Can you work these out from the model? Positions are in its coordinate system, mm. A direction names the side the tool comes from. Round coordinates to 2 decimals unless told otherwise and drop trailing zeros.
from build123d import *

# Parameters (mm, degrees)
SKETCH1_W           = 38
SKETCH1_H           = 70
BOSS_EXTRUDE1_DEPTH = 5
SKETCH2_R           = 1.65
CUT_EXTRUDE1_DEPTH  = 134.018795664
FILLET1_R           = 3
FILLET2_DEPTH       = 5
SKETCH3_W           = 188
SKETCH3_H           = 3
BOSS_EXTRUDE2_DEPTH = 8
SKETCH4_W           = 5
SKETCH4_H           = 39
BOSS_EXTRUDE3_DEPTH = 8
BOSS_EXTRUDE4_DEPTH = 5
FILLET3_SIZE        = 40
FILLET3_SIZE_2      = 10
FILLET4_SIZE        = 40
FILLET4_SIZE_2      = 10
CUT_EXTRUDE2_DEPTH  = 134.165310942


with BuildPart() as part:
    # Sketch1 → Boss-Extrude1 (new body)
    with BuildSketch(Plane.XY):
        with Locations((19, -35)):
            Rectangle(SKETCH1_W, SKETCH1_H)
        Polygon((-75, 15), (-75, 0), (0, 0), (38, 0), (113, 0), (113, 15), align=None)
    extrude(amount=BOSS_EXTRUDE1_DEPTH)

    # Sketch2 → Cut-Extrude1 (cut, through all)
    with BuildSketch(Plane.XY.offset(5)):
        with Locations((34, -66)):
            Circle(SKETCH2_R)
        with Locations((4, -66)):
            Circle(SKETCH2_R)
        with Locations((4, -40)):
            Circle(SKETCH2_R)
        with Locations((34, -40)):
            Circle(SKETCH2_R)
    extrude(amount=-CUT_EXTRUDE1_DEPTH, mode=Mode.SUBTRACT)

    # Fillet1
    fillet1_edges = [part.edges().sort_by_distance(p)[0] for p in [
        (38, -70, 2.5),
        (0, -70, 2.5),
    ]]
    fillet(fillet1_edges, radius=FILLET1_R)

    # Fillet2: read off the stored shape, not the designer's step
    # Fillet2 outline → Fillet2 (add)
    with BuildSketch(Plane.XY):
        with BuildLine():
            add(Edge.make_bspline(
                [(58, 0), (38, 0), (38, -20)],
                knots=[0, 0, 0, 1, 1, 1], degree=2, weights=[1, 0.052631579, 1]))
            Line((58, 0), (38, 0))
            Line((38, 0), (38, -20))
        make_face()
        with BuildLine():
            Line((0, 0), (-20, 0))
            add(Edge.make_bspline(
                [(-20, 0), (0, 0), (0, -20)],
                knots=[0, 0, 0, 1, 1, 1], degree=2, weights=[1, 0.052631579, 1]))
            Line((0, -20), (0, 0))
        make_face()
    extrude(amount=FILLET2_DEPTH)

    # Sketch3 → Boss-Extrude2 (add)
    with BuildSketch(Plane.XY.offset(5)):
        with Locations((19, 4.5)):
            Rectangle(SKETCH3_W, SKETCH3_H)
    extrude(amount=BOSS_EXTRUDE2_DEPTH)

    # Sketch4 → Boss-Extrude3 (add)
    with BuildSketch(Plane.XY.offset(5)):
        with Locations((19, -16.5)):
            Rectangle(SKETCH4_W, SKETCH4_H)
    extrude(amount=BOSS_EXTRUDE3_DEPTH)

    # Sketch5 → Boss-Extrude4 (add)
    with BuildSketch(Plane.XY.offset(5)):
        Polygon((-52, 0), (-57.902965871, 0), (-60, 0), (0, -30), (0, -25), align=None)
        Polygon((38, -30), (98, 0), (90, 0), (38, -25), align=None)
    extrude(amount=-BOSS_EXTRUDE4_DEPTH)

    # Fillet3
    # a fillet whose section is not a circle: 40, 10 mm, written as the material it takes off along each edge
    with BuildSketch(Plane(origin=(-75, 15, -100), x_dir=(1, 0, 0), z_dir=(0, 0, 1))) as fillet3_piece_1:
        with BuildLine():
            Bezier((FILLET3_SIZE, 0), (0, 0), (0, -FILLET3_SIZE_2), weights=[1, 0.707106781, 1])
            Line((0, -FILLET3_SIZE_2), (0, 0))
            Line((0, 0), (FILLET3_SIZE, 0))
        make_face()
    extrude(amount=205, mode=Mode.SUBTRACT)

    # Fillet4
    # a fillet whose section is not a circle: 40, 10 mm, written as the material it takes off along each edge
    with BuildSketch(Plane(origin=(113, 15, -100), x_dir=(-1, 0, 0), z_dir=(0, 0, 1))) as fillet4_piece_1:
        with BuildLine():
            Bezier((FILLET4_SIZE, 0), (0, 0), (0, FILLET4_SIZE_2), weights=[1, 0.707106781, 1])
            Line((0, FILLET4_SIZE_2), (0, 0))
            Line((0, 0), (FILLET4_SIZE, 0))
        make_face()
    extrude(amount=205, mode=Mode.SUBTRACT)

    # Sketch6 → Cut-Extrude2 (cut, through all)
    with BuildSketch(Plane.XY.offset(5)):
        with BuildLine():
            Line((3.671572875, -13.862410437), (-3.399494937, -6.791342626))
            ThreePointArc((-3.399494937, -6.791342626), (-3.399494937, -1.134488376), (2.257359313, -1.134488376))
            Line((2.257359313, -1.134488376), (9.328427125, -8.205556188))
            ThreePointArc((9.328427125, -8.205556188), (9.328427125, -13.862410437), (3.671572875, -13.862410437))
        make_face()
        with BuildLine():
            Line((28.671572875, -8.445013015), (35.742640687, -1.373945203))
            ThreePointArc((35.742640687, -1.373945203), (41.399494937, -1.373945203), (41.399494937, -7.030799453))
            Line((41.399494937, -7.030799453), (34.328427125, -14.101867265))
            ThreePointArc((34.328427125, -14.101867265), (28.671572875, -14.101867265), (28.671572875, -8.445013015))
        make_face()
    extrude(amount=-CUT_EXTRUDE2_DEPTH, mode=Mode.SUBTRACT)


solid = part.part
(1) If I drill on line 1 (X direction, y = -66, z = 3.7); line 2 (Y direction, x = 34, z = 2.35); line 3 (Y direction, x = 4, z = 1.45), over which ranges is the centre line in solid material (lowest first)?
Worked answers:
line 1: x = 0 to 2.35, 5.65 to 32.35, 35.65 to 38
line 2: y = -70 to -67.65, -64.35 to -41.65, -38.35 to -14.4, -3.12 to 15
line 3: y = -70 to -67.65, -64.35 to -41.65, -38.35 to -14.16, -2.88 to 15
(2) Will these pins go through, and if not, where does the flat tip stop? P1, Ø6, axis at y = -59, z = 3, coming from the +X side; P2, Ø4, axis at x = -38, z = 3.5, coming from the -Y side; P3, Ø4, axis at x = 42.5, z = 7.5, coming from the +Y side.
Worked answers:
P1: stops at x = 38
P2: stops at y = -12
P3: stops at y = 6
(3) If we mould it in two halves opening along Y, with no side actions, what happens to faces 1 (the flat face through (38, -49, 2)), 2 (the flat face through (68, -15, 3)), 3 (the flat face through (37.91, -10.52, 2.54))? For each: released by +Y, released by -Y, zero draft, split by the parting line, or undercut.
Worked answers:
face 1: zero draft
face 2: released by -Y
face 3: undercut
(4) For faces 4 (the flat face through (-30, 3, 9)), 5 (the flat face through (32.158, -4.959, 2.535)), 6 (the flat face through (21.5, -17, 9)), which set-ups out of +Z, -Z, +X, -X, +Y, -Y let a thin tool reach every point of the face, with its end or its side?
Worked answers:
face 4: +Z, -X, -Y
face 5: +Z, -Z
face 6: +Z, +X, -Y
